Build history of the part. All positions in model axes, mm. Face numbers are marked on the shaded views. Coordinates: 2 decimals unless noted, no trailing zeros. Write each loop counter-clockwise with the first axis right and the second up, starting at its lowest first coordinate (ties: lowest second). Pieces come first, ordered by that corner, then holes. Notation, with made-up numbers: (33.5, -15.5) -> (40.5, -15.5) arc R34 ccw to (40.5, 18.5) -> close; hole circle Ø5 at (55.25, -3.5). An arc over 180 degrees is marked (long way). Write each question's results on one line, items separated by ' | '. Start each with the question number.
Q1. Saw through at C-C on x = 57.5. Give the cut face in (y, z), and give its area (3 significant figures).
Q2. Drop flat-ended pins along their axis: pin 1 Ø10 at (x, z) = (-10, 18) entering from +Y; pin 2 Ø2.5 at (x, z) = (22.66, 6.25) entering from -Y; pin 3 Ø1.5 at (y, z) = (22.5, -3.5) entering from +X; pin 4 Ø1.5 at (x, y) = (19.5, 16.5) entering from -Z. Give the stop position or say it passes through.
Q3. Saw through at D-D on z = -5.5. Give the cut face in (x, y), and give its area (3 significant figures).
Q4. Drill centre lines: line 1 (X direction, y = 11, z = 6.25); line 2 (X direction, y = 7.5, z = 7.5); line 3 (Y direction, x = -7.5, z = 13.5). Where is each one in solid material? Low to high.
Q5. Saw through at A-A on z = 6.25. Give the cut face in (x, y).
Q6. Two-plate mould, pull along Z, no slides. Class the marked faces 1, 2 and 3: released by +Z, released by -Z, zero draft, split by the parting line, or undercut.
Q7. Saw through at B-B on y = 3.75. Give the cut face in (x, z).
from build123d import *

# Parameters (mm, degrees)
SKETCH1_R           = 5
SKETCH1_R_2         = 1.5
BOSS_EXTRUDE2_DEPTH = 26
SKETCH2_R           = 6.25
BOSS_EXTRUDE3_DEPTH = 2
CUT_EXTRUDE1_START  = -2
SKETCH3_R           = 5
CUT_EXTRUDE1_DEPTH  = 2


with BuildPart() as part:
    # Sketch1 → Boss-Extrude2 (new body)
    with BuildSketch(Plane(origin=(0, 0, 0), x_dir=(1, 0, 0), z_dir=(0, 1, 0))):
        with BuildLine():
            Line((-19.568980619, 0), (53.439105934, 9.332584612))
            ThreePointArc((53.439105934, 9.332584612), (71.14040073, -6.25), (53.439105934, -21.832584612))
            Line((53.439105934, -21.832584612), (-19.568980619, -12.5))
            ThreePointArc((-19.568980619, -12.5), (-25.818980619, -6.25), (-19.568980619, 0))
        make_face()
        with Locations(Location((-19.568980619, -6.25, 0), (0, 0, 90))):
            Circle(SKETCH1_R, mode=Mode.SUBTRACT)
        with Locations(Location((22.660710056, -6.25, 0), (0, 0, 90))):
            Circle(SKETCH1_R_2, mode=Mode.SUBTRACT)
    extrude(amount=BOSS_EXTRUDE2_DEPTH)

    # Sketch2 → Boss-Extrude3 (add)
    with BuildSketch(Plane(origin=(0, 26, 0), x_dir=(1, 0, 0), z_dir=(0, 1, 0))):
        with Locations(Location((-19.568980619, -6.25, 0), (0, 0, 270))):
            Circle(SKETCH2_R)
    extrude(amount=BOSS_EXTRUDE3_DEPTH)

    # Sketch3 → Cut-Extrude1 (cut)
    with BuildSketch(Plane(origin=(0, 28, 0), x_dir=(1, 0, 0), z_dir=(0, 1, 0)).offset(CUT_EXTRUDE1_START)):
        with Locations(Location((-19.568980619, -6.25, 0), (0, 0, 90))):
            Circle(SKETCH3_R)
    extrude(amount=CUT_EXTRUDE1_DEPTH, mode=Mode.SUBTRACT)


solid = part.part
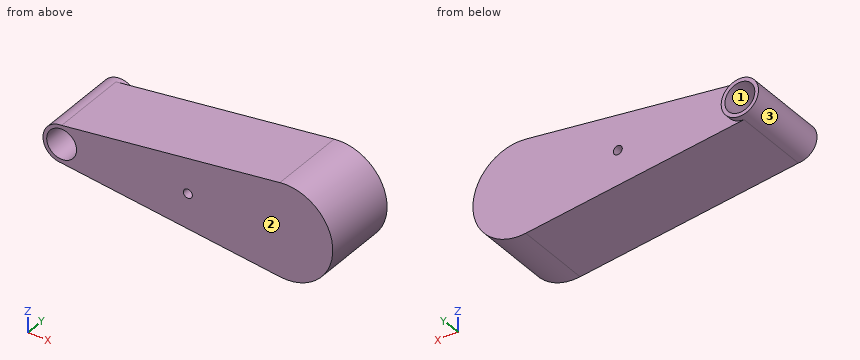
Returned:
1) outline: (0, -9.32) -> (26, -9.32) -> (26, 21.82) -> (0, 21.82) -> close | area: 810 mm2
2) pin 1: stops at y = 26 | pin 2: passes through | pin 3: stops at x = 68.31 | pin 4: stops at z = -5.09
3) outline: (23.46, 0) -> (65.86, 0) -> (65.86, 26) -> (23.46, 26) -> close | area: 1,100 mm2
4) line 1: x = -25.82 to -24.57, -14.57 to 21.16, 24.16 to 71.14 | line 2: x = -25.69 to -24.41, -14.73 to 21.83, 23.49 to 71.09 | line 3: y = 0 to 26
5) outline: (-25.82, 0) -> (-24.57, 0) -> (-24.57, 28) -> (-25.82, 28) -> close; (-14.57, 0) -> (21.16, 0) -> (21.16, 26) -> (-13.32, 26) -> (-13.32, 28) -> (-14.57, 28) -> close; (24.16, 0) -> (71.14, 0) -> (71.14, 26) -> (24.16, 26) -> close
6) face 1: undercut | face 2: zero draft | face 3: split by the parting line
7) outline: (-19.57, 0) -> (53.44, -9.33) arc R15.71 ccw (long way) to (53.44, 21.83) -> (-19.57, 12.5) arc R6.25 ccw to start; hole circle Ø10 at (-19.57, 6.25); hole circle Ø3 at (22.66, 6.25)
